```python
from build123d import *

# Parameters (mm, degrees)
SKETCH1_W           = 24.765
SKETCH1_H           = 25.4
SKETCH1_W_2         = 25.4
SKETCH1_H_2         = 24.765
BOSS_EXTRUDE1_DEPTH = 10.16
SKETCH2_W           = 20.32
SKETCH2_H           = 20.32
SKETCH2_H_2         = 22.225
SKETCH2_W_2         = 22.225
CUT_EXTRUDE1_DEPTH  = 10.16
SKETCH4_W           = 20.32
SKETCH4_H           = 2.54
SKETCH4_W_2         = 2.54
SKETCH4_H_2         = 20.32
CUT_EXTRUDE2_DEPTH  = 5.08
BOSS_EXTRUDE2_DEPTH = 1.27
SKETCH6_R           = 1.27
CUT_EXTRUDE3_DEPTH  = 1.27


with BuildPart() as part:
    # Sketch1 → Boss-Extrude1 (new body)
    with BuildSketch(Plane.XY):
        with Locations((-25.0825, 0)):
            Rectangle(SKETCH1_W, SKETCH1_H)
        Rectangle(SKETCH1_W_2, SKETCH1_H)
        with Locations((0, 25.0825)):
            Rectangle(SKETCH1_W_2, SKETCH1_H_2)
        with Locations((25.0825, 0)):
            Rectangle(SKETCH1_W, SKETCH1_H)
        with Locations((0, -25.0825)):
            Rectangle(SKETCH1_W_2, SKETCH1_H_2)
    extrude(amount=BOSS_EXTRUDE1_DEPTH)

    # Sketch2 → Cut-Extrude1 (cut)
    with BuildSketch(Plane.XY.offset(10.16)):
        Rectangle(SKETCH2_W, SKETCH2_H)
        with Locations((0, 23.8125)):
            Rectangle(SKETCH2_W, SKETCH2_H_2)
        with Locations((0, -23.8125)):
            Rectangle(SKETCH2_W, SKETCH2_H_2)
        with Locations((-23.8125, 0)):
            Rectangle(SKETCH2_W_2, SKETCH2_H)
        with Locations((23.8125, 0)):
            Rectangle(SKETCH2_W_2, SKETCH2_H)
    extrude(amount=-CUT_EXTRUDE1_DEPTH, mode=Mode.SUBTRACT)

    # Sketch4 → Cut-Extrude2 (cut)
    with BuildSketch(Plane.XY.offset(10.16)):
        with Locations((0, 36.195)):
            Rectangle(SKETCH4_W, SKETCH4_H)
        with Locations((36.195, 0)):
            Rectangle(SKETCH4_W_2, SKETCH4_H_2)
        with Locations((-36.195, 0)):
            Rectangle(SKETCH4_W_2, SKETCH4_H_2)
        with Locations((0, -36.195)):
            Rectangle(SKETCH4_W, SKETCH4_H)
    extrude(amount=-CUT_EXTRUDE2_DEPTH, mode=Mode.SUBTRACT)

    # Sketch5 → Boss-Extrude2 (add)
    with BuildSketch(Plane.XY):
        Polygon((-37.465, 12.7), (-12.7, 37.465), (-12.7, 12.7), align=None)
        Polygon((12.7, 37.465), (37.465, 12.7), (12.7, 12.7), align=None)
        Polygon((37.465, -12.7), (12.7, -12.7), (12.7, -37.465), align=None)
        Polygon((-12.7, -37.465), (-12.7, -12.7), (-37.465, -12.7), align=None)
    extrude(amount=BOSS_EXTRUDE2_DEPTH)

    # Sketch6 → Cut-Extrude3 (cut)
    with BuildSketch(Plane.XY.offset(1.27)):
        with Locations((-20.425141584, 20.425141584)):
            Circle(SKETCH6_R)
        with Locations((20.425141584, 20.425141584)):
            Circle(SKETCH6_R)
        with Locations(Location((20.425141584, -20.425141584, 0), (0, 0, 180))):
            Circle(SKETCH6_R)
        with Locations(Location((-20.425141584, -20.425141584, 0), (0, 0, 180))):
            Circle(SKETCH6_R)
    extrude(amount=-CUT_EXTRUDE3_DEPTH, mode=Mode.SUBTRACT)


solid = part.part
```
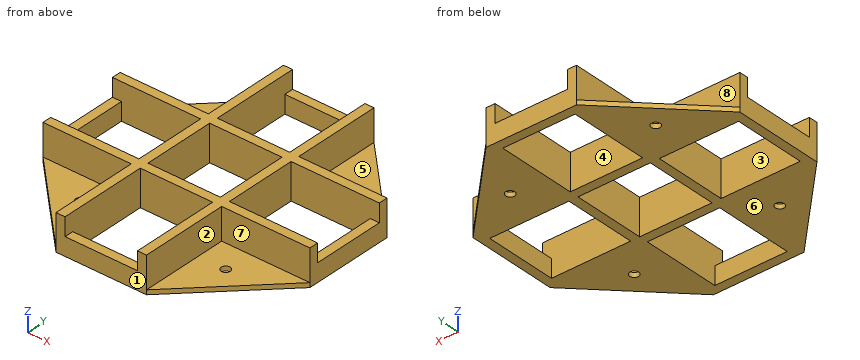
Part model, mm, in its own coordinate system. Face numbers are marked on the shaded views. A direction names the side the tool comes from. Coordinates: 2 decimals unless noted, no trailing zeros. Order: outer loops, then holes, each group sorted by start corner. A loop starts at its lowest first (then second) coordinate and runs counter-clockwise, first axis right, second up. Notation, with made-up numbers: (-4.5, -27) - (10.5, -27) arc R15 cw to (10.5, -5) - close; hole circle Ø9 at (48.5, 25). An arc over 180 degrees is marked (long way). Return JSON: item names as keys, results as strings. Group by question number.
Item 1: Pin check, flat tips, straight feed: pin 1 (4 mm diameter, centred on x = -22, z = 7, fed in from -Y); pin 2 (1 mm diameter, centred on y = -23.5, z = 2, fed in from -X); pin 3 (0.8 mm diameter, centred on x = 36.5, y = -2.5, fed in from +Z). Stop position of each tip, or through.
Item 2: Cut at D-D (y = -24). List the corners of the cut face in (x, z) (3 decimals), plus the area to 3 significant figures.
Item 3: Drill centre lines: probe 1 along Y at (x, z) = (8, 1) (3 decimals); probe 2 along X at (y, z) = (-25, 5.25). Where is each one in solid material? Low to high. Write a range as from..to.
Item 4: Which spindle directions (+Z, -Z, +X, -X, +Y, -Y) get a long thin tool onto all of the face, cutting with end or side? Do the marked faces 4, 5, 6, 7 and 8. Say none if no direction does.
Item 5: Cut at A-A (y = -3). List the corners of the cut face in (x, z) (3 decimals).
Item 6: Pull direction X, two halves, no side cores. Call the marked faces 1, 2 and 3: pulls with the +X half, pulls with the -X half, needs draft (parallel to the pull), parting line crosses it, or undercut.
Check values:
{
 "1": {"pin 1": "stops at y = -12.7", "pin 2": "stops at x = -12.7", "pin 3": "stops at z = 5.08"},
 "2": {"outline": "(-26.165, 0) - (-10.16, 0) - (-10.16, 10.16) - (-12.7, 10.16) - (-12.7, 1.27) - (-26.165, 1.27) - close; (10.16, 0) - (26.165, 0) - (26.165, 1.27) - (12.7, 1.27) - (12.7, 10.16) - (10.16, 10.16) - close", "area": "85.8 mm2"},
 "3": {"probe 1": "y = -37.465..-34.925, -12.7..-10.16, 10.16..12.7, 34.925..37.465", "probe 2": "x = -12.7..-10.16, 10.16..12.7"},
 "4": {"face 4": "+Z, -Z", "face 5": "+Z, +X, +Y", "face 6": "-Z, +X, -X, +Y, -Y", "face 7": "+Z, +X, -Y", "face 8": "+Z, -X, +Y"},
 "5": {"outline": "(-37.465, 0) - (-34.925, 0) - (-34.925, 5.08) - (-37.465, 5.08) - close; (-12.7, 0) - (-10.16, 0) - (-10.16, 10.16) - (-12.7, 10.16) - close; (10.16, 0) - (12.7, 0) - (12.7, 10.16) - (10.16, 10.16) - close; (34.925, 0) - (37.465, 0) - (37.465, 5.08) - (34.925, 5.08) - close"},
 "6": {"face 1": "needs draft", "face 2": "pulls with the +X half", "face 3": "undercut"}
}
